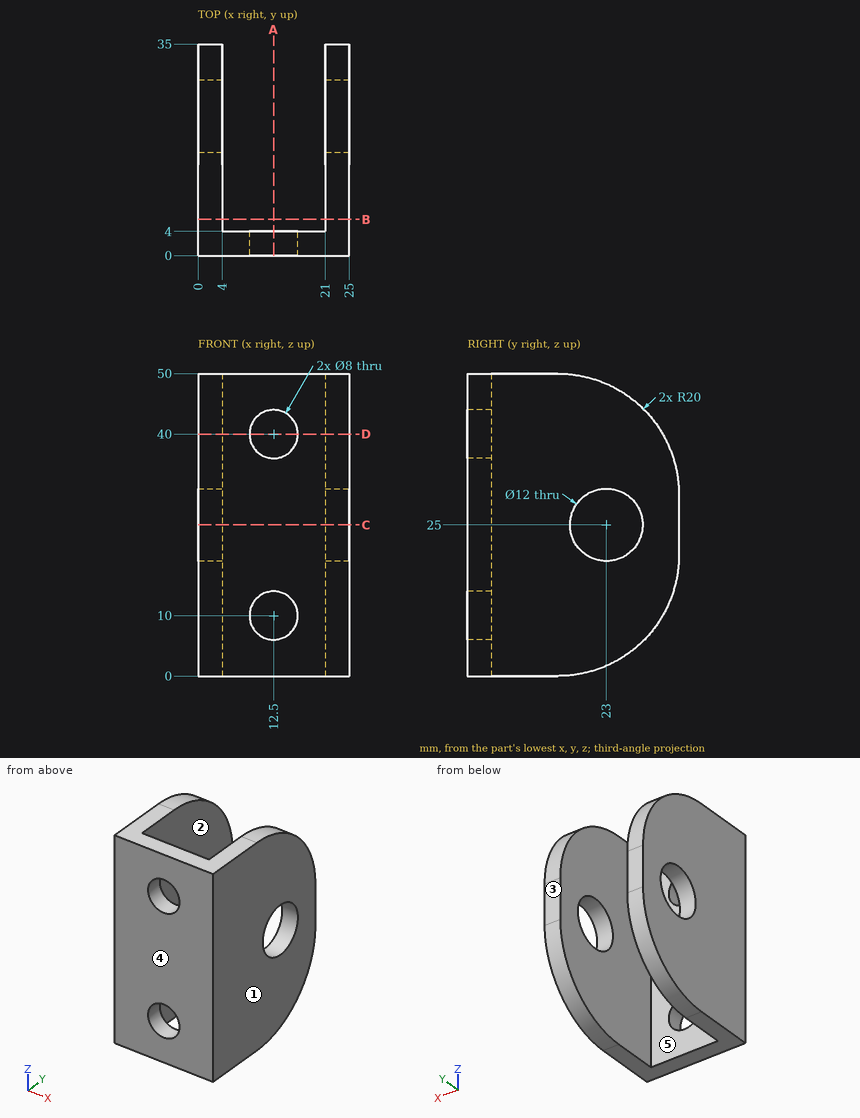
Can you work these out from the drawing? Everything is in mm from the part's minimum corner. A direction names the side the tool comes from. Coordinates: 2 decimals unless noted, no trailing zeros. Write each loop counter-clockwise with the first axis right and the second up, starting at its lowest first coordinate (ties: lowest second). Pieces come first, ordered by that corner, then holes. Notation, with made-up numbers: (-11, 77) -> (9, 77) arc R24 ccw to (9, 112) -> close; hole circle Ø6 at (13, 23). An arc over 180 degrees is marked (long way). Write item = value, one per line.
(1) Imagine slicing it at A-A (x = 12.5). Please give me the cut outline in (y, z).
Verdict:
outline = (0, 0) -> (4, 0) -> (4, 6) -> (0, 6) -> close; (0, 14) -> (4, 14) -> (4, 36) -> (0, 36) -> close; (0, 44) -> (4, 44) -> (4, 50) -> (0, 50) -> close
(2) Imagine slicing it at C-C (z = 25). Please give me the cut outline in (x, y), and give its area (3 significant figures).
Verdict:
outline = (0, 0) -> (25, 0) -> (25, 17) -> (21, 17) -> (21, 4) -> (4, 4) -> (4, 17) -> (0, 17) -> close; (0, 29) -> (4, 29) -> (4, 35) -> (0, 35) -> close; (21, 29) -> (25, 29) -> (25, 35) -> (21, 35) -> close
area = 252 mm^2
(3) For pin 1 (2 mm diameter, centred on x = 18.5, z = 38.5, fed in from +Y), with a flat end and sliding along its axis, tell me the tip position at first contact or that it passes through.
Verdict:
pin_1 = 4
(4) On a 3-axis mill with a long thin cutter (end or side, diameter ignored), from which of +Z, -Z, +X, -X, +Y, -Y can I reach the whole of each face in a straight line? I mean the marked faces 4 and 5. Say none if no direction works.
Verdict:
face_4 = +Z, -Z, +X, -X, -Y
face_5 = +Z, -Z, +Y
(5) Imagine slicing it at D-D (z = 40). Please give me the cut outline in (x, y).
Verdict:
outline = (0, 0) -> (8.5, 0) -> (8.5, 4) -> (4, 4) -> (4, 32.32) -> (0, 32.32) -> close; (16.5, 0) -> (25, 0) -> (25, 32.32) -> (21, 32.32) -> (21, 4) -> (16.5, 4) -> close
(6) If I drill on probe 1 along Z at (x, y) = (12.5, 1.65); probe 2 along X at (y, z) = (18.5, 41.5); probe 3 along Y at (x, z) = (23.9, 25), over which ranges is the centre line in solid material (lowest first)?
Verdict:
probe_1 = 0 to 6, 14 to 36, 44 to 50
probe_2 = 0 to 4, 21 to 25
probe_3 = 0 to 17, 29 to 35
(7) Thinking about a two-plate mould opening in X: for the marked faces 1, 2 and 3, which applies, +X half, -X half, draft (parallel to the pull), parting line (faces both ways), or undercut?
Verdict:
face_1 = +X half
face_2 = undercut
face_3 = draft
(8) Imagine slicing it at B-B (y = 6). Please give me the cut outline in (x, z), and give its area (3 significant figures).
Verdict:
outline = (0, 0) -> (4, 0) -> (4, 50) -> (0, 50) -> close; (21, 0) -> (25, 0) -> (25, 50) -> (21, 50) -> close
area = 400 mm^2
